Source: CAD feature listing. Evaluate the final solid. Frame: model axes, mm. Give positions to 0.01 mm unless a question says otherwise; leave off trailing zeros. Loops run counter-clockwise (first coordinate to the right, second up) from the corner with the lowest first, then second, coordinate; pieces in that order, holes last. Notation, with made-up numbers: (56, 88) -> (100, 88) arc R36 cw to (100, 126) -> close; hole circle Ø11 at (66, -2). An arc over 180 degrees is marked (long way). Put each result on its own line as item: value.
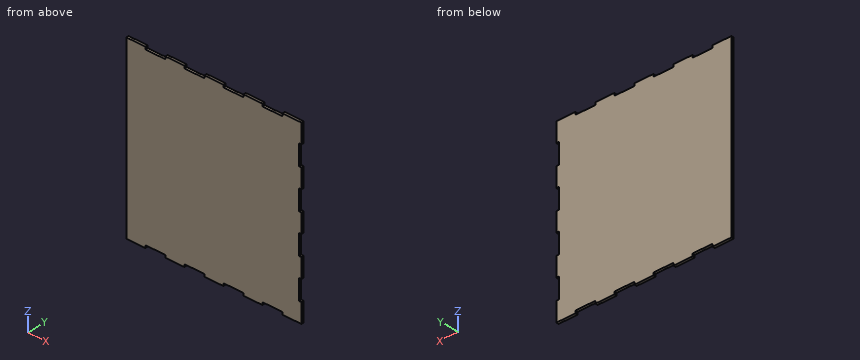
```python
from build123d import *

# Parameters (mm, degrees)
SKIZZE1_W                       = 350
SKIZZE1_H                       = 350
GRUNDPLATTE_DEPTH               = 5
SKIZZE2_W                       = 40
SKIZZE2_H                       = 5
SCHNITT_LINEAR_AUSTRAGEN1_DEPTH = 6
KREISMUSTER1_COUNT              = 2
KREISMUSTER1_ANGLE              = 90


with BuildPart() as part:
    # Skizze1 → Grundplatte (new body)
    with BuildSketch(Plane(origin=(0, 0, 0), x_dir=(1, 0, 0), z_dir=(0, 1, 0))):
        Rectangle(SKIZZE1_W, SKIZZE1_H)
    extrude(amount=GRUNDPLATTE_DEPTH)

    # Skizze2 → Schnitt-Linear austragen1 (cut, through all)
    with BuildSketch(Plane(origin=(0, 5, 0), x_dir=(1, 0, 0), z_dir=(0, 1, 0))):
        with Locations((-117, 172.5)):
            Rectangle(SKIZZE2_W, SKIZZE2_H)
        with Locations((-39, 172.5)):
            Rectangle(SKIZZE2_W, SKIZZE2_H)
        with Locations((39, 172.5)):
            Rectangle(SKIZZE2_W, SKIZZE2_H)
        with Locations((117, 172.5)):
            Rectangle(SKIZZE2_W, SKIZZE2_H)
    schnitt_linear_austragen1 = extrude(amount=-SCHNITT_LINEAR_AUSTRAGEN1_DEPTH, mode=Mode.SUBTRACT)

    # Spiegeln1: Schnitt-Linear austragen1 across plane
    add(schnitt_linear_austragen1.mirror(Plane.XY), mode=Mode.SUBTRACT)

    # Kreismuster1: Schnitt-Linear austragen1 ×2 about axis
    kreismuster1_axis = Axis((0, 0, 0), (0, -1, 0))
    for i in range(1, KREISMUSTER1_COUNT):
        add(schnitt_linear_austragen1.rotate(kreismuster1_axis, i * KREISMUSTER1_ANGLE / (KREISMUSTER1_COUNT - 1)), mode=Mode.SUBTRACT)


solid = part.part
```
(1) Line query: probe 1 along Z at (x, y) = (-44.5, 2.05); probe 2 along X at (y, z) = (0.45, 134.5). Output: solid intervals per line, ascending. Write a range as from..to.
Calculated:
probe 1: z = -170..170
probe 2: x = -175..170
(2) First-contact query: P1, Ø2.5, axis at y = 2, z = -36.5, coming from the +X side; P2, Ø1.5, axis at x = 119, y = 1.5, coming from the -Z side. Flat tips, straight axial feed; report the tip coordinate or a pass-through.
Calculated:
P1: stops at x = 170
P2: stops at z = -170
(3) Section A-A on x = 115.5. Return loops of the section in (y, z), then the cut area to 3 significant figures.
Calculated:
outline: (0, -170) -> (5, -170) -> (5, 170) -> (0, 170) -> close
area: 1,700 mm²
